Could you check a few things on this model? Use its own coordinates, in mm. A direction names the side the tool comes from. Give positions to 0.01 mm unless a question says otherwise; leave off trailing zeros. Order: outer loops, then holes, each group sorted by start corner. A loop starts at its lowest first (then second) coordinate and runs counter-clockwise, first axis right, second up. Notation, with made-up numbers: M 17.25,-2 L 36.25,-2 A17 ccw 36.25,22 Z; hole C -24.75,4.25 d5. An arc over 180 degrees is marked long. Use a Markdown table: item, result. Add a question column.
Item 1: Suppose I cut it at C-C on y = 8. Write out the boundary of the cut face in (x, z), plus the area to 3 significant figures.
Item 2: Suppose I cut it at D-D on x = 6.25. Write out the boundary of the cut face in (y, z), plus the area to 3 significant figures.
Item 3: If I drill on L1, parallel to Z at x = 0, y = 9.1; L2, parallel to X at y = 9.25, z = 0, over which ranges is the centre line in solid material (lowest first)? Write a range as from..to.
Item 4: Suppose I cut it at A-A on x = 0. Write out the boundary of the cut face in (y, z), plus the area to 3 significant figures.
Item 5: Suppose I cut it at B-B on z = 0. Write out the boundary of the cut face in (x, y), plus the area to 3 significant figures.
Item 6: I'm going to push flat-ended pins straight in: pin 1 Ø1.5 at (y, z) = (7, 2.5) entering from +X; pin 2 Ø3 at (y, z) = (10.5, 5) entering from +X; pin 3 Ø1 at (x, y) = (-10, 9.5) entering from -Z. Where does each tip first touch, or does it pass through?
Item 7: For faces 1 (the face through (8.7, 7.8, 7.7)), 2 (the face through (-11.3, 9.5, 0.7)), 3 (the face through (-0.1, 8.9, -11.1)), which set-ups out of +Z, -Z, +X, -X, +Y, -Y let a thin tool reach every point of the face, with its end or its side?
from build123d import *

# Parameters (mm, degrees)
SKETCH1_R               = 10.95
SKETCH1_R_2             = 6.05
BOSS_EXTRUDE1_DEPTH     = 2
BOSS_EXTRUDE2_START     = 12
SKETCH1_3_R             = 10.95
SKETCH1_3_R_2           = 6.05
BOSS_EXTRUDE2_DEPTH     = 12
BOSS_EXTRUDE3_START     = -2.5
SKETCH2_R               = 12.95
SKETCH2_R_2             = 10.95
BOSS_EXTRUDE3_DEPTH     = 11.5
CUT_EXTRUDE1_DEPTH      = 22.895319134
CUT_EXTRUDE1_DEPTH_BACK = 22.895319134
SKETCH3_W               = 100
SKETCH3_H               = 23
CUT_EXTRUDE3_DEPTH      = 22.07018035
CUT_EXTRUDE3_DEPTH_BACK = 22.07018035
BOSS_EXTRUDE4_START     = 12
SKETCH1_5_R             = 10.95
SKETCH1_5_R_2           = 6.05
BOSS_EXTRUDE4_DEPTH     = 12
CHAMFER1_SIZE           = 1
BOSS_EXTRUDE5_START     = 12
SKETCH7_R               = 6.05
BOSS_EXTRUDE5_DEPTH     = 12
CUT_EXTRUDE5_DEPTH      = 22.07018035
CUT_EXTRUDE5_DEPTH_BACK = 22.07018035
SKETCH6_R               = 3.25
CUT_EXTRUDE7_START      = -8
CUT_EXTRUDE7_DEPTH      = 8


with BuildPart() as part:
    # Sketch1 → Boss-Extrude1 (new body)
    # profile 1 of 2: a face of its own
    with BuildSketch(Plane(origin=(0, 0, 0), x_dir=(1, 0, 0), z_dir=(0, 1, 0))):
        with Locations(Location((0, 0, 0), (0, 0, 270))):
            Circle(SKETCH1_R)
        Circle(SKETCH1_R_2, mode=Mode.SUBTRACT)
    # profile 2 of 2: a face of its own
    with BuildSketch(Plane(origin=(0, 0, 0), x_dir=(1, 0, 0), z_dir=(0, 1, 0))):
        Circle(SKETCH1_R_2)
    extrude(amount=-BOSS_EXTRUDE1_DEPTH)

    # Sketch1<3> → Boss-Extrude2 (add)
    with BuildSketch(Plane(origin=(0, 0, 0), x_dir=(1, 0, 0), z_dir=(0, 1, 0)).offset(BOSS_EXTRUDE2_START)):
        with Locations(Location((0, 0, 0), (0, 0, 270))):
            Circle(SKETCH1_3_R)
        with Locations(Location((0, 0, 0), (0, 0, 270))):
            Circle(SKETCH1_3_R_2, mode=Mode.SUBTRACT)
    extrude(amount=-BOSS_EXTRUDE2_DEPTH)

    # Sketch2 → Boss-Extrude3 (add)
    with BuildSketch(Plane(origin=(0, 12, 0), x_dir=(1, 0, 0), z_dir=(0, 1, 0)).offset(BOSS_EXTRUDE3_START)):
        with Locations(Location((0, 0, 0), (0, 0, 270))):
            Circle(SKETCH2_R)
        with Locations(Location((0, 0, 0), (0, 0, 270))):
            Circle(SKETCH2_R_2, mode=Mode.SUBTRACT)
    extrude(amount=-BOSS_EXTRUDE3_DEPTH)

    # Sketch3 → Cut-Extrude1 (cut, two sides: drawn at the far end of the back side and taken through both)
    with BuildSketch(Plane(origin=(0, 0, 0), x_dir=(1, 0, 0), z_dir=(0, 1, 0)).offset(-CUT_EXTRUDE1_DEPTH_BACK)):
        with Locations((0, -23)):
            Rectangle(SKETCH3_W, SKETCH3_H)
        with Locations((0, 23)):
            Rectangle(SKETCH3_W, SKETCH3_H)
    extrude(amount=CUT_EXTRUDE1_DEPTH + CUT_EXTRUDE1_DEPTH_BACK, mode=Mode.SUBTRACT)

    # Sketch4 → Cut-Extrude3 (cut, two sides: drawn at the far end of the back side and taken through both)
    with BuildSketch(Plane.XY.offset(-CUT_EXTRUDE3_DEPTH_BACK)):
        Polygon((13, 12), (4.5, 12), (13, 3.5), align=None)
    extrude(amount=CUT_EXTRUDE3_DEPTH + CUT_EXTRUDE3_DEPTH_BACK, mode=Mode.SUBTRACT)

    # Sketch1<5> → Boss-Extrude4 (add)
    with BuildSketch(Plane(origin=(0, 0, 0), x_dir=(1, 0, 0), z_dir=(0, 1, 0)).offset(BOSS_EXTRUDE4_START)):
        with Locations(Location((0, 0, 0), (0, 0, 270))):
            Circle(SKETCH1_5_R)
        with Locations(Location((0, 0, 0), (0, 0, 270))):
            Circle(SKETCH1_5_R_2, mode=Mode.SUBTRACT)
    extrude(amount=-BOSS_EXTRUDE4_DEPTH)

    # Chamfer1
    # the kernel refuses this chamfer: 1 mm, written as the material it takes off along each edge
    with BuildSketch(Plane(origin=(8.525883186, 9.5, 11.5), x_dir=(0, 0.027495876610585647, -0.9996219169112968), z_dir=(-1, 0, 0))) as chamfer1_piece_1_section:
        Polygon((CHAMFER1_SIZE * 0.999621916911, CHAMFER1_SIZE * 0.0274958766106), (-CHAMFER1_SIZE * 0.0274958766106, CHAMFER1_SIZE * 0.999621916911), (0, 0), align=None)
    chamfer1_piece_1 = extrude(amount=17.051766372, mode=Mode.PRIVATE)
    chamfer1_piece_1 = chamfer1_piece_1 - Plane(origin=(0, 9.159933663, 0), x_dir=(0, 0, 1), z_dir=(0, 1, 0)) * Cylinder(10.95, 39, mode=Mode.PRIVATE)
    add(chamfer1_piece_1, mode=Mode.SUBTRACT)
    with BuildSketch(Plane(origin=(8.525883186, 9.5, -11.5), x_dir=(0, 0.027495876610585647, 0.9996219169112968), z_dir=(-1, 0, 0))) as chamfer1_piece_2_section:
        Polygon((CHAMFER1_SIZE * 0.999621916911, -CHAMFER1_SIZE * 0.0274958766106), (-CHAMFER1_SIZE * 0.0274958766106, -CHAMFER1_SIZE * 0.999621916911), (0, 0), align=None)
    chamfer1_piece_2 = extrude(amount=17.051766372, mode=Mode.PRIVATE)
    chamfer1_piece_2 = chamfer1_piece_2 - Plane(origin=(0, 9.159933662, 0), x_dir=(0, 0, 1), z_dir=(0, 1, 0)) * Cylinder(10.95, 39, mode=Mode.PRIVATE)
    add(chamfer1_piece_2, mode=Mode.SUBTRACT)

    # Sketch7 → Boss-Extrude5 (add)
    with BuildSketch(Plane(origin=(0, 0, 0), x_dir=(1, 0, 0), z_dir=(0, 1, 0)).offset(BOSS_EXTRUDE5_START)):
        Circle(SKETCH7_R)
    extrude(amount=-BOSS_EXTRUDE5_DEPTH)

    # Sketch6 → Cut-Extrude5 (cut, two sides: drawn at the far end of the back side and taken through both)
    with BuildSketch(Plane(origin=(0, 0, 0), x_dir=(1, 0, 0), z_dir=(0, 1, 0)).offset(-CUT_EXTRUDE5_DEPTH_BACK)):
        with Locations(Location((0, 0, 0), (0, 0, 270))):
            Circle(SKETCH6_R)
    extrude(amount=CUT_EXTRUDE5_DEPTH + CUT_EXTRUDE5_DEPTH_BACK, mode=Mode.SUBTRACT)

    # Sketch9 → Cut-Extrude7 (cut)
    with BuildSketch(Plane.XZ.offset(2).offset(CUT_EXTRUDE7_START)):
        with BuildLine():
            Line((5.954200198, 11.5), (-5.954200198, 11.5))
            ThreePointArc((-5.954200198, 11.5), (-12.95, 0), (-5.954200198, -11.5))
            Line((-5.954200198, -11.5), (5.954200198, -11.5))
            ThreePointArc((5.954200198, -11.5), (12.95, 0), (5.954200198, 11.5))
        make_face()
    extrude(amount=CUT_EXTRUDE7_DEPTH, mode=Mode.SUBTRACT)


solid = part.part
Findings below:
| question | item | result |
|---|---|---|
| 1 | outline | M -5.95,-11.5 L 5.95,-11.5 A12.95 ccw 8.5,-9.77 L 8.5,-6.9 A10.95 ccw 8.5,6.9 L 8.5,9.77 A12.95 ccw 5.95,11.5 L -5.95,11.5 A12.95 ccw Z; hole C 0,0 d6.5 |
| 1 | area | 433 mm^2 |
| 2 | outline | M 6,-11.34 L 8.66,-11.34 L 9.5,-10.5 L 9.5,-8.99 L 12,-8.99 L 12,8.99 L 9.5,8.99 L 9.5,10.5 L 8.66,11.34 L 6,11.34 Z |
| 2 | area | 124 mm^2 |
| 3 | L1 | z = -10.95..-3.25, 3.25..10.95 |
| 3 | L2 | x = -12.95..-3.25, 3.25..10.95 |
| 4 | outline | M 6,-11.5 L 8.5,-11.5 L 9.05,-10.95 L 12,-10.95 L 12,-3.25 L 6,-3.25 Z; M 6,3.25 L 12,3.25 L 12,10.95 L 9.05,10.95 L 8.5,11.5 L 6,11.5 Z |
| 4 | area | 95.5 mm^2 |
| 5 | outline | M -12.95,6 L -3.25,6 L -3.25,12 L -10.95,12 L -10.95,9.5 L -12.95,9.5 Z; M 3.25,6 L 10.95,6 L 10.95,12 L 3.25,12 Z |
| 5 | area | 99.4 mm^2 |
| 6 | pin 1 | stops at x = 10.81 |
| 6 | pin 2 | stops at x = 10.38 |
| 6 | pin 3 | stops at z = -8.8 |
| 7 | face 1 | +Z, +X, +Y |
| 7 | face 2 | -X, +Y |
| 7 | face 3 | -Z, +Y |
